Check sheet for the modelled part. Datum: model origin and axes. Units: mm. Face numbers are marked on the shaded views. Give positions to 0.01 mm unless a question says otherwise; leave off trailing zeros. Order: outer loops, then holes, each group sorted by start corner. A loop starts at its lowest first (then second) coordinate and runs counter-clockwise, first axis right, second up.
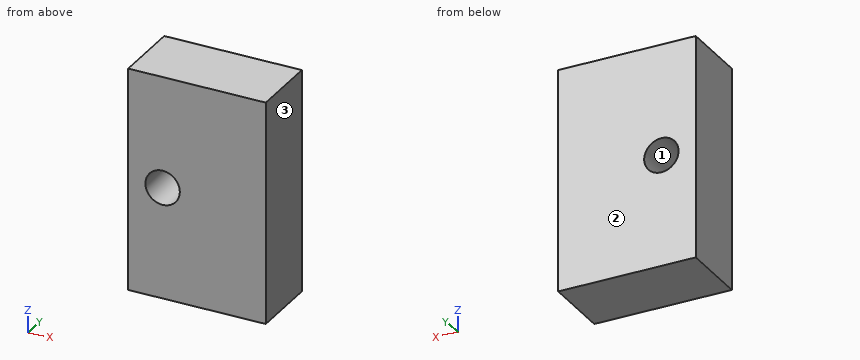
Autodesk Inventor part; units mm, degrees
ref_plane "YZ Plane" through (0, 0, 0) normal (1, 0, 0) x (0, 1, 0)
ref_plane "XZ Plane" through (0, 0, 0) normal (0, 1, 0) x (-1, 0, 0)
ref_plane "XY Plane" through (0, 0, 0) normal (0, 0, 1) x (1, 0, 0)
sketch "Sketch1" plane through (0, 0, 0) normal (0, 1, 0) x (-1, 0, 0)
  line L0 (-25.4, 41.0981) -> (25.4, 41.0981)
  line L1 (25.4, 41.0981) -> (25.4, -41.0981)
  line L2 (25.4, -41.0981) -> (-25.4, -41.0981)
  line L3 (-25.4, -41.0981) -> (-25.4, 41.0981)
  line L4 (-25.4, 41.0981) -> (25.4, -41.0981) construction
  line L5 (25.4, 41.0981) -> (-25.4, -41.0981) construction
  circle A0 centre (12.7, 0) radius 6.35
  line L6 (0, 0) -> (12.7, 0) construction
  dimension "d0" = 50.8
  dimension "d1" = 82.1961
  dimension "d2" = 12.7
  dimension "d3" = 12.7
extrude "Extrusion1" add sketch "Sketch1" along normal blind 25.4
properties part number "Motor Black Box" material "Stainless Steel"
(1) Release check for a two-part mould opening along X. For the marked faces 1, 2 and 3 record: released by +X, released by -X, zero draft, split by the parting line, or undercut.
Response values:
face 1: undercut
face 2: zero draft
face 3: released by +X
(2) Cross-section at A-A on z = 0. Enter the section's corners in (x, y).
Response values:
outline: (-25.4, 0) - (-19.05, 0) - (-19.05, 25.4) - (-25.4, 25.4) - close; (-6.35, 0) - (25.4, 0) - (25.4, 25.4) - (-6.35, 25.4) - close
(3) Material ranges on L1, parallel to Z at x = -12.7, y = 19.5; L2, parallel to Z at x = -8.5, y = 24; L3, parallel to X at y = 3.75, z = -3, recorded low to high.
Response values:
L1: z = -41.1 to -6.35, 6.35 to 41.1
L2: z = -41.1 to -4.76, 4.76 to 41.1
L3: x = -25.4 to -18.3, -7.1 to 25.4
(4) Cross-section at B-B on x = -12.7. Enter the section's corners in (y, z).
Response values:
outline: (0, -41.1) - (25.4, -41.1) - (25.4, -6.35) - (0, -6.35) - close; (0, 6.35) - (25.4, 6.35) - (25.4, 41.1) - (0, 41.1) - close
(5) Cross-section at C-C on y = 11. Enter the section's corners in (x, z), then the cut area to 3 significant figures.
Response values:
outline: (-25.4, -41.1) - (25.4, -41.1) - (25.4, 41.1) - (-25.4, 41.1) - close; hole circle Ø12.7 at (-12.7, 0)
area: 4,050 mm2
